Check sheet for the modelled part. Datum: model origin and axes. Units: mm. A direction names the side the tool comes from. Round coordinates to 2 decimals unless told otherwise and drop trailing zeros. Write each loop counter-clockwise with the first axis right and the second up, starting at its lowest first coordinate (ties: lowest second). Pieces come first, ordered by that corner, then holes. Notation, with made-up numbers: M 2.25,-3.75 L 32.25,-3.75 A18 cw 32.25,17.25 Z; hole C 75.25,-37 d1. An arc over 180 degrees is marked long. Answer in a Markdown table with one row per item.
Autodesk Inventor part; units mm, degrees
ref_plane "YZ Plane" through (0, 0, 0) normal (1, 0, 0) x (0, 1, 0)
ref_plane "XZ Plane" through (0, 0, 0) normal (0, 1, 0) x (-1, 0, 0)
ref_plane "XY Plane" through (0, 0, 0) normal (0, 0, 1) x (1, 0, 0)
sketch "Sketch1" plane through (0, 0, 0) normal (0, 1, 0) x (-1, 0, 0)
  circle A0 centre (0, 0) radius 11.43
  circle A1 centre (0, 0) radius 9.525
  dimension "d0" = 22.86
  dimension "d1" = 19.05
extrude "Extrusion1" add sketch "Sketch1" along normal blind 6.35
sketch "Sketch2" plane through (0, 6.35, 0) normal (0, 1, 0) x (1, 0, 0)
  circle A0 centre (0, 0) radius 11.43
extrude "Extrusion2" add sketch "Sketch2" along normal blind 3.175
sketch "Sketch3" plane through (0, 9.525, 0) normal (0, 1, 0) x (1, 0, 0)
  circle A0 centre (0, 0) radius 1.1
  dimension "d6" = 2.2
extrude "Extrusion3" cut sketch "Sketch3" against normal blind 7.9375
sketch "Sketch6" plane through (0, 0, 0) normal (0, -1, 0) x (1, 0, 0)
  line L0 (-16.0948, 0) -> (0, 0)
  line L1 (0, 0) -> (0, -15.3841)
  line L2 (0, -15.3841) -> (-16.0948, -15.3841)
  line L3 (-16.0948, -15.3841) -> (-16.0948, 0)
  line L4 (-16.0948, 14.6504) -> (12.3807, 14.6504)
  line L5 (12.3807, 14.6504) -> (12.3807, -15.3841)
  line L6 (12.3807, -15.3841) -> (-16.0948, -15.3841)
  line L7 (-16.0948, -15.3841) -> (-16.0948, 14.6504)
extrude "Extrusion6" cut sketch "Sketch6" against normal blind 6.35 contours L7 L4 L5 L6 L1 L0
sketch "Sketch7" plane through (0, 0, -9.525) normal (1, 0, 0) x (0, 0, -1)
  line L0 (1.905, 6.35) -> (-20.955, 6.35)
  line L1 (1.905, 6.35) -> (0, 6.35)
  line L2 (0, 6.35) -> (0, 0)
  line L3 (0, 0) -> (1.905, 0)
  line L4 (1.905, 0) -> (1.905, 6.35)
  point P0 (-9.525, 0)
  point P1 (-9.525, 6.35)
extrude "Extrusion7" add sketch "Sketch7" along normal blind 11.43
sketch "Sketch8" plane through (0, 0, 0) normal (0, -1, 0) x (1, 0, 0)
  line L0 (0, 0) -> (-10.5625, -10.5625)
  line L1 (0, 0) -> (14.9376, 0) construction
  line L2 (-10.5625, -10.5625) -> (-17.6997, 3.3244)
  line L3 (-17.6997, 3.3244) -> (0, 0)
  dimension "d18" = 135
extrude "Extrusion8" cut sketch "Sketch8" against normal blind 6.35
sketch "Sketch9" plane through (0, 0, 0) normal (0, -1, 0) x (1, 0, 0)
  line L0 (0, 0) -> (-6.0166, -14.5254)
  line L1 (0, 0) -> (15.7222, 0) construction
  line L2 (-6.0166, -14.5254) -> (-13.1372, -7.2627)
  line L3 (-13.1372, -7.2627) -> (0, 0)
  dimension "d21" = 112.5
extrude "Extrusion9" cut sketch "Sketch9" against normal blind 6.35
sketch "Sketch13" plane through (0, 9.525, 0) normal (0, 1, 0) x (1, 0, 0)
  line L0 (0, 0) -> (-53.8815, 53.8815)
  line L1 (0, 0) -> (76.2, 0) construction
  circle A0 centre (-53.8815, 53.8815) radius 10.16
  arc A1 (6.3182, 9.525) -> (0, 11.43) centre (0, 0) ccw
  line L2 (0, 11.43) -> (0, 53.8815)
  line L3 (0, 53.8815) -> (-50.1886, 63.3466)
  arc A2 (-4.3741, 10.5599) -> (6.3182, 9.525) centre (0, 0) ccw
  line L4 (-11.43, 0) -> (-11.43, 42.4515)
  line L5 (-11.43, 42.4515) -> (-43.7215, 53.8815)
  circle A3 centre (-53.8815, 53.8815) radius 1.65
  circle A4 centre (0, 0) radius 1.1
  circle A5 centre (0, 0) radius 1.65
  dimension "d44" = 76.2
  dimension "d45" = 135
  dimension "d46" = 20.32
  dimension "d47" = 100.68
  dimension "d48" = 3.3
  dimension "d49" = 3.3
extrude "Extrusion13" add sketch "Sketch13" against normal blind 3.175 contours A2 L4 L0 | L0 L4 L5 A0 L3 L2 A1 A2 | A0
fillet "Fillet3" radius 50.8 1 edges at (-11.43, 7.9375, -42.4515)
fillet "Fillet4" radius 7.62 1 edges at (-43.7215, 7.9375, -53.8815)
fillet "Fillet5" radius 63.5 1 edges at (0, 7.9375, -53.8815)
mirror "Mirror1" about plane through (0, 6.35, -11.43) normal (0, 1, 0) of "Extrusion1", "Extrusion7"
sketch "Sketch14" plane through (0, 12.7, -11.43) normal (0, 1, 0) x (1, 0, 0)
  line L0 (0, -11.43) -> (-4.3741, -0.8701)
  line L1 (-4.3741, -0.8701) -> (-16.9777, -0.8701)
  line L2 (-16.9777, -0.8701) -> (-16.9777, -27.9599)
  line L3 (-16.9777, -27.9599) -> (23.6628, -27.9599)
  line L4 (0, -1.905) -> (11.43, -1.905)
  line L5 (23.6628, -27.9599) -> (11.43, -1.905)
  line L6 (11.43, -1.905) -> (0, -1.905)
  line L7 (0, -1.905) -> (0, -11.43)
extrude "Extrusion14" cut sketch "Sketch14" against normal blind 3.175
sketch "Sketch15" plane through (0, 6.35, 0) normal (0, -1, 0) x (1, 0, 0)
  line L0 (-24.6585, 25.4032) -> (37.4015, 25.4032)
  line L1 (37.4015, 25.4032) -> (37.4015, -39.3047)
  line L2 (37.4015, -39.3047) -> (-24.6585, -39.3047)
  line L3 (-24.6585, -39.3047) -> (-24.6585, 25.4032)
  point P0 (0, 0)
extrude "Extrusion15" cut sketch "Sketch15" along normal blind 26.9875
1. Draft check along X on faces 1 (the face through (3, 12.7, -10)), 2 (the face through (1.05, 7.96, -0.33)), 3 (the face through (-11.43, 8, -3)). Enter one of: +X half, -X half, draft (parallel to the pull), parting line (faces both ways), or undercut.
Found:
| item | result |
|---|---|
| face 1 | draft |
| face 2 | undercut |
| face 3 | -X half |
2. Go/stop test with flat-tipped pins: pin 1 (1.9 mm diameter, centred on x = 4.5, y = 10.5, fed in from -Z); pin 2 (22.5 mm diameter, centred on x = -22, z = -10.5, fed in from +Y) (3 decimals); pin 3 (1 mm diameter, centred on y = 7.5, z = -2, fed in from -X). Record where each tip stops, or that it passes through.
Found:
| item | result |
|---|---|
| pin 1 | stops at z = -11.43 |
| pin 2 | stops at y = 9.525 |
| pin 3 | stops at x = -11.43 |
3. Access from +Z, -Z, +X, -X, +Y, -Y to the whole of each face (thin tool, end or side, straight path). Record for faces 4 (the face through (6, 9, -11.43)), 5 (the face through (-2.199, 11.135, -11.216)), 6 (the face through (-4.004, 11.135, -9.668)), 7 (the face through (-1.833, 11.135, -9.347)), 8 (the face through (-17.7, 7.96, -31.02)).
Found:
| item | result |
|---|---|
| face 4 | -Z, +X, +Y, -Y |
| face 5 | -Z, -X, +Y |
| face 6 | +Z, -X, +Y |
| face 7 | +Z, +X, +Y |
| face 8 | +Z, +Y, -Y |
4. Scan lines: L1, parallel to X at y = 8.7, z = 0; L2, parallel to Y at x = -12, z = -37.5 (3 decimals); L3, parallel to Z at x = -55, y = 8.25. Record each from-to range of solid material in increasing order.
Found:
| item | result |
|---|---|
| L1 | x = -11.43 to -1.1, 1.1 to 11.43 |
| L2 | y = 6.35 to 9.525 |
| L3 | z = -63.98 to -55.09, -52.67 to -43.78 |
5. Section check A-A, the plane y = 10.5. Record the cut outline in (x, z) (3 decimals), and give its area (3 significant figures).
Found:
| item | result |
|---|---|
| outline | M -4.374,-10.56 A11.43 ccw 0,-11.43 L 11.43,-11.43 L 11.43,-9.525 L 0,-9.525 A9.525 cw -3.645,-8.8 Z |
| area | 29.6 mm2 |
6. Section check C-C, the plane z = -17. Record the cut outline in (x, y) (3 decimals).
Found:
| item | result |
|---|---|
| outline | M -12.512,6.35 L -1.179,6.35 L -1.179,9.525 L -12.512,9.525 Z |
7. Section check B-B, the plane x = -9.5. Record the cut outline in (y, z) (3 decimals), and give its area (3 significant figures).
Found:
| item | result |
|---|---|
| outline | M 6.35,-35.823 L 9.525,-35.823 L 9.525,6.356 L 6.35,6.356 Z |
| area | 134 mm2 |
